from build123d import *

# Parameters (mm, degrees)
SKETCH1_R                       = 7.5
SKETCH1_R_2                     = 3
BOSS_EXTRUDE1_DEPTH             = 7.5
SKETCH2_R                       = 7.5
SKETCH2_R_2                     = 3
BOSS_EXTRUDE2_DEPTH             = 1
SKETCH3_R                       = 7.5
SKETCH3_R_2                     = 4
BOSS_EXTRUDE3_DEPTH             = 3
SKETCH4_R                       = 7.5
SKETCH4_R_2                     = 5.075
BOSS_EXTRUDE4_DEPTH             = 4.1
SKETCH5_R                       = 7.5
SKETCH5_R_2                     = 4
BOSS_EXTRUDE5_DEPTH             = 3.1
CBORE_FOR_M3_SBHCS1_D           = 3.2
CBORE_FOR_M3_SBHCS1_DEPTH       = 10
CBORE_FOR_M3_SBHCS1_CBORE_D     = 6.7
CBORE_FOR_M3_SBHCS1_CBORE_DEPTH = 1.65
CBORE_FOR_M3_SBHCS1_TIP         = 0.96137699
SKETCH9_W                       = 15
SKETCH9_H                       = 25.2
CUT_EXTRUDE2_DEPTH              = 8.5000001
FILLET1_R                       = 1
FILLET2_R                       = 2


with BuildPart() as part:
    # Sketch1 → Boss-Extrude1 (new body, symmetric)
    with BuildSketch(Plane.XY):
        Circle(SKETCH1_R)
        Circle(SKETCH1_R_2, mode=Mode.SUBTRACT)
    extrude(amount=BOSS_EXTRUDE1_DEPTH, both=True)

    # Sketch2 → Boss-Extrude2 (add)
    with BuildSketch(Plane.XY.offset(7.5)):
        Circle(SKETCH2_R)
        Circle(SKETCH2_R_2, mode=Mode.SUBTRACT)
    extrude(amount=-BOSS_EXTRUDE2_DEPTH)

    # Sketch3 → Boss-Extrude3 (add)
    with BuildSketch(Plane.XY.offset(7.5)):
        Circle(SKETCH3_R)
        Circle(SKETCH3_R_2, mode=Mode.SUBTRACT)
    extrude(amount=BOSS_EXTRUDE3_DEPTH)

    # Sketch4 → Boss-Extrude4 (add)
    with BuildSketch(Plane.XY.offset(10.5)):
        Circle(SKETCH4_R)
        Circle(SKETCH4_R_2, mode=Mode.SUBTRACT)
    extrude(amount=BOSS_EXTRUDE4_DEPTH)

    # Sketch5 → Boss-Extrude5 (add)
    with BuildSketch(Plane.XY.offset(14.6)):
        Circle(SKETCH5_R)
        Circle(SKETCH5_R_2, mode=Mode.SUBTRACT)
    extrude(amount=BOSS_EXTRUDE5_DEPTH)

    # CBORE for M3 SBHCS1
    with Locations(Plane(origin=(0, 7.5, 0), x_dir=(1, 0, 0), z_dir=(0, 1, 0))):
        with Locations((0, 1.5)):
            CounterBoreHole(CBORE_FOR_M3_SBHCS1_D / 2, CBORE_FOR_M3_SBHCS1_CBORE_D / 2, CBORE_FOR_M3_SBHCS1_CBORE_DEPTH, depth=CBORE_FOR_M3_SBHCS1_DEPTH)
            with Locations((0, 0, -(CBORE_FOR_M3_SBHCS1_DEPTH + CBORE_FOR_M3_SBHCS1_TIP / 2))):  # 118° drill point
                Cone(0, CBORE_FOR_M3_SBHCS1_D / 2, CBORE_FOR_M3_SBHCS1_TIP, mode=Mode.SUBTRACT)

    # Sketch9 → Cut-Extrude2 (cut, through all)
    with BuildSketch(Plane(origin=(0, 0, 0), x_dir=(1, 0, 0), z_dir=(0, 1, 0))):
        with Locations((0, -5.1)):
            Rectangle(SKETCH9_W, SKETCH9_H)
    extrude(amount=-CUT_EXTRUDE2_DEPTH, mode=Mode.SUBTRACT)

    # Fillet1
    fillet1_edges = [part.edges().sort_by_distance(p)[0] for p in [
        (0, 4, 17.7),
    ]]
    fillet(fillet1_edges, radius=FILLET1_R)

    # Fillet2
    fillet2_edges = [part.edges().sort_by_distance(p)[0] for p in [
        (0, 3, -7.5),
    ]]
    fillet(fillet2_edges, radius=FILLET2_R)


solid = part.part
Read the model definition and answer for the solid it produces. Units are mm, in the model's axes. A direction names the side the tool comes from. Coordinates: 2 decimals unless noted, no trailing zeros. Loops run counter-clockwise (first coordinate to the right, second up) from the corner with the lowest first, then second, coordinate; pieces in that order, holes last. Notation, with made-up numbers: (6, 76.5) -> (23, 76.5) arc R30 ccw to (23, 102.5) -> close; hole circle Ø3 at (30, 1.5). An arc over 180 degrees is marked (long way). Answer in a Markdown table with one row per item.
Item 1: Each of these flat-tipped pins is pushed along its axis until it touches: P1, Ø1, axis at y = 5.5, z = 1.5, coming from the +X side; P2, Ø5, axis at x = 0, z = -1.5, coming from the +Y side; P3, Ø3, axis at y = 4.5, z = 14, coming from the +X side. Where does it stop, or does it pass through?
Returned:
| item | result |
|---|---|
| P1 | stops at x = 5.59 |
| P2 | stops at y = 5.85 |
| P3 | stops at x = 6.87 |
Item 2: A cutting plane is placed at D-D on z = 16. Determine the outline of the cut face in (x, y).
Returned:
| item | result |
|---|---|
| outline | (-7.5, 0) -> (-4, 0) arc R4 cw to (4, 0) -> (7.5, 0) arc R7.5 ccw to start |
Item 3: A cutting plane is placed at A-A on x = 0. Determine the outline of the cut face in (y, z) (3 decimals).
Returned:
| item | result |
|---|---|
| outline | (3, -5.5) arc R2 ccw to (5, -7.5) -> (7.5, -7.5) -> (7.5, -4.85) -> (5.85, -4.85) -> (5.85, -3.1) -> (3, -3.1) -> close; (3, 0.1) -> (5.85, 0.1) -> (5.85, 1.85) -> (7.5, 1.85) -> (7.5, 17.7) -> (5, 17.7) arc R1 ccw to (4, 16.7) -> (4, 14.6) -> (5.075, 14.6) -> (5.075, 10.5) -> (4, 10.5) -> (4, 7.5) -> (3, 7.5) -> close |
Item 4: For faces 1 (the cylindrical face through (0, 3, 1)), 2 (the flat face through (1, 5.85, 0)), 3 (the cylindrical face through (0, 4, 16)), 4 (the flat face through (5, 0, 5)), 5 (the flat face through (0, 4.2, 14.6)), determine the directions among +Z, -Z, +X, -X, +Y, -Y from which every point of the face is accessible in a straight line to the end or side of a thin tool.
Returned:
| item | result |
|---|---|
| face 1 | +Z, -Z, -Y |
| face 2 | +Y |
| face 3 | +Z, -Y |
| face 4 | +Z, -Z, +X, -X, -Y |
| face 5 | -Y |
Item 5: For a pull along Z with two mould halves and no side action, classify faces 6 (the flat face through (-0.1, 5.5, -7.5)), 7 (the cylindrical face through (0, 4, 9)), 8 (the cylindrical face through (-1.48, 4.17, -0.89)), 9 (the flat face through (-0.1, 5.5, 17.7)) as released by +Z, released by -Z, zero draft, split by the parting line, or undercut.
Returned:
| item | result |
|---|---|
| face 6 | released by -Z |
| face 7 | zero draft |
| face 8 | undercut |
| face 9 | released by +Z |
Item 6: A cutting plane is placed at B-B on z = -1.5. Determine the outline of the cut face in (x, y).
Returned:
| item | result |
|---|---|
| outline | (-7.5, 0) -> (-3, 0) arc R3 cw to (-1.6, 2.54) -> (-1.6, 5.85) -> (-3.35, 5.85) -> (-3.35, 6.71) arc R7.5 ccw to start; (1.6, 2.54) arc R3 cw to (3, 0) -> (7.5, 0) arc R7.5 ccw to (3.35, 6.71) -> (3.35, 5.85) -> (1.6, 5.85) -> close |
Item 7: Straight lines are drawn through the part: line 1 along Z through (x, y) = (0, 6.85); line 2 along X through (y, z) = (3.75, -1.25); line 3 along Z through (x, y) = (0, 4.5). For each, find the intervals that lie inside material, in ascending order. Write a range as [from, to].
Returned:
| item | result |
|---|---|
| line 1 | z = [-7.5, -4.85], [1.85, 17.7] |
| line 2 | x = [-6.5, -1.58], [1.58, 6.5] |
| line 3 | z = [-7.44, -3.1], [0.1, 10.5], [14.6, 17.57] |
Item 8: A cutting plane is placed at C-C on z = 3.75. Determine the outline of the cut face in (x, y).
Returned:
| item | result |
|---|---|
| outline | (-7.5, 0) -> (-3, 0) arc R3 cw to (3, 0) -> (7.5, 0) arc R7.5 ccw to start |
